```python
from build123d import *

# Parameters (mm, degrees)
BOSS_EXTRUDE2_DEPTH      = 0.79375
FILLET2_R                = 0.396875
CIRPATTERN5_COUNT        = 4
FILLET2_OF_CIRPATTERN5_R = 0.396875


with BuildPart() as part:
    # Sketch3 → Revolve2 (revolve)
    with BuildSketch(Plane(origin=(0, 0, 0), x_dir=(0, 0, -1), z_dir=(1, 0, 0)), mode=Mode.PRIVATE) as revolve2_sk:
        with BuildLine():
            Line((0, 0.79375), (0, 0))
            Line((0, 0), (127, 0))
            Line((127, 0), (127, 3.175))
            Line((127, 3.175), (69.85, 11.752276451))
            ThreePointArc((69.85, 11.752276451), (63.517656161, 12.462740177), (57.15, 12.7))
            Line((57.15, 12.7), (38.1, 12.7))
            ThreePointArc((38.1, 12.7), (18.1414881, 9.65411308), (0, 0.79375))
        make_face()
    revolve(revolve2_sk.sketch.rotate(Axis((0, 0, 0), (0, 0, -1)), 90), axis=Axis((0, 0, 0), (0, 0, -1)))

    # Sketch5 → Boss-Extrude2 (add, symmetric)
    with BuildSketch(Plane(origin=(0, 0, 0), x_dir=(0, 0, -1), z_dir=(1, 0, 0))):
        Polygon((120.65, 19.05), (127, 19.05), (127, 0), (88.9, 6.35), align=None)
    boss_extrude2 = extrude(amount=BOSS_EXTRUDE2_DEPTH, both=True)

    # Fillet2
    fillet2_edges = [part.edges().sort_by_distance(p)[0] for p in [
        (-0.79375, 19.05, -123.825),
        (0.79375, 19.05, -123.825),
        (-0.79375, 13.61067, -107.051675),
        (0.79375, 13.61067, -107.051675),
    ]]
    fillet(fillet2_edges, radius=FILLET2_R)

    # CirPattern5: Boss-Extrude2 ×4 about axis
    cirpattern5_axis = Axis((0, 0, 0), (0, 0, 1))
    for i in range(1, CIRPATTERN5_COUNT):
        add(boss_extrude2.rotate(cirpattern5_axis, i * 360 / CIRPATTERN5_COUNT))

    # Fillet2 of CirPattern5
    fillet2_of_cirpattern5_edges = [part.edges().sort_by_distance(p)[0] for p in [
        (-19.05, -0.79375, -123.825),
        (-19.05, 0.79375, -123.825),
        (-13.61067, -0.79375, -107.051675),
        (-13.61067, 0.79375, -107.051675),
        (0.79375, -19.05, -123.825),
        (-0.79375, -19.05, -123.825),
        (0.79375, -13.61067, -107.051675),
        (-0.79375, -13.61067, -107.051675),
        (19.05, 0.79375, -123.825),
        (19.05, -0.79375, -123.825),
        (13.61067, 0.79375, -107.051675),
        (13.61067, -0.79375, -107.051675),
    ]]
    fillet(fillet2_of_cirpattern5_edges, radius=FILLET2_OF_CIRPATTERN5_R)


solid = part.part
```
Geometry: final body of the model. Coordinates: model frame, mm. A direction names the side the tool comes from. Round coordinates to 2 decimals unless told otherwise and drop trailing zeros. Order: outer loops, then holes, each group sorted by start corner. A loop starts at its lowest first (then second) coordinate and runs counter-clockwise, first axis right, second up. Notation, with made-up numbers: M 79.25,18.5 L 87.25,18.5 A20 ccw 87.25,31.5 Z; hole C -29,-18 d6. An arc over 180 degrees is marked long. Use one line per item in the form item = value. Start each with the question number.
Q1. Cut plane B-B (z = -86). Return loops of the section in (x, y), and give its area (3 significant figures).
Q2. Mould query, pull axis Z, two halves, no side actions, for faces 1 (the face through (13.545, -0.006, -106.888)), 2 (the face through (0.674, 13.592, -107.309)), 3 (the face through (0, 0, -127)), 4 (the face through (-10.1, 7.7, -47.5)). Classes: +Z half, -Z half, draft (parallel to the pull), parting line (faces both ways), or undercut.
Q3. Pin query (flat end, axial travel): pin 1 Ø8 at (x, z) = (-7.5, -114.5) entering from +Y; pin 2 Ø2 at (x, y) = (1, -3) entering from +Z; pin 3 Ø2 at (y, z) = (-4.5, -111.5) entering from -X; pin 4 Ø4 at (x, y) = (-12.5, -9.5) entering from +Z. Return the tip coordinate at first contact, or that it passes through.
Q4. Access query for faces 5 (the face through (0.794, -11, -114)), 6 (the face through (-0.681, -13.586, -107.311)), 7 (the face through (-0.794, 11, -114)), 8 (the face through (13.592, 0.674, -107.309)), 9 (the face through (0.674, -13.592, -107.309)). Directions: +Z, -Z, +X, -X, +Y, -Y. A direction counts if a zero-diameter tool reaches every point of the face in a straight line with its end or side. Return the directions, or none.
Q5. Material intervals for line 1 (Z direction, x = -0.5, y = -4.5) (3 decimals); line 2 (X direction, y = -6, z = -102); line 3 (X direction, y = 3.5, z = -21), sorted ascending. Write a range as [from, to].
Q6. Cut plane A-A (z = -47). Return loops of the section in (x, y), and give its area (3 significant figures).
Geometry results:
q1.outline = C 0,0 d18.66
q1.area = 273 mm^2
q2.face_1 = undercut
q2.face_2 = undercut
q2.face_3 = -Z half
q2.face_4 = draft
q3.pin_1 = 3.73
q3.pin_2 = -2.06
q3.pin_3 = -4.27
q3.pin_4 = through
q4.face_5 = -Z, +X, -Y
q4.face_6 = -X, -Y
q4.face_7 = -Z, -X, +Y
q4.face_8 = +X, +Y
q4.face_9 = +X, -Y
q5.line_1 = [-127, -6.055]
q5.line_2 = [-3.46, 3.46]
q5.line_3 = [-9.88, 9.88]
q6.outline = C 0,0 d25.4
q6.area = 507 mm^2
